Design review of the part shown in the three views and the two pictorial views. Dimensions are in mm from the part's minimum x, y and z. Coordinates: 2 decimals unless noted, no trailing zeros. Write each loop counter-clockwise with the first axis right and the second up, starting at its lowest first coordinate (ties: lowest second). Pieces come first, ordered by that corner, then holes. Notation, with made-up numbers: (81, 12.5) - (125, 12.5) arc R26 cw to (125, 51.5) - close; hole circle Ø2 at (31, 11.5). An arc over 180 degrees is marked (long way). Return JSON: item names as keys, results as strings. Group by question number.
(1) We need section D-D on y = 76. State the section outline as (x, z) points.
(2) Draft analysis for pull direction X (two halves, no side actions). For the marked faces 1, 2 and 3, state which applies: released by +X, released by -X, zero draft, split by the parting line, or undercut.
(3) For pin 1 Ø17.5 at (x, y) = (44.5, 55) entering from +Z; pin 2 Ø1.5 at (y, z) = (42, 2.5) entering from -X; pin 3 Ø5 at (y, z) = (69, 8.5) entering from +X (1 decimal); pin 4 Ø1.5 at (y, z) = (68, 2) entering from +X, all flat-tipped, find the tip position at first contact; note any pin that passes through.
(4) To check wall thickness, follow L1, parallel to Y at x = 44.45, z = 17.2 (1 decimal); L2, parallel to Y at x = 44.45, z = 8.75; L3, parallel to X at y = 32, z = 15. State the ranges of each line that lie inside material, in increasing order. Write a range as from..to.
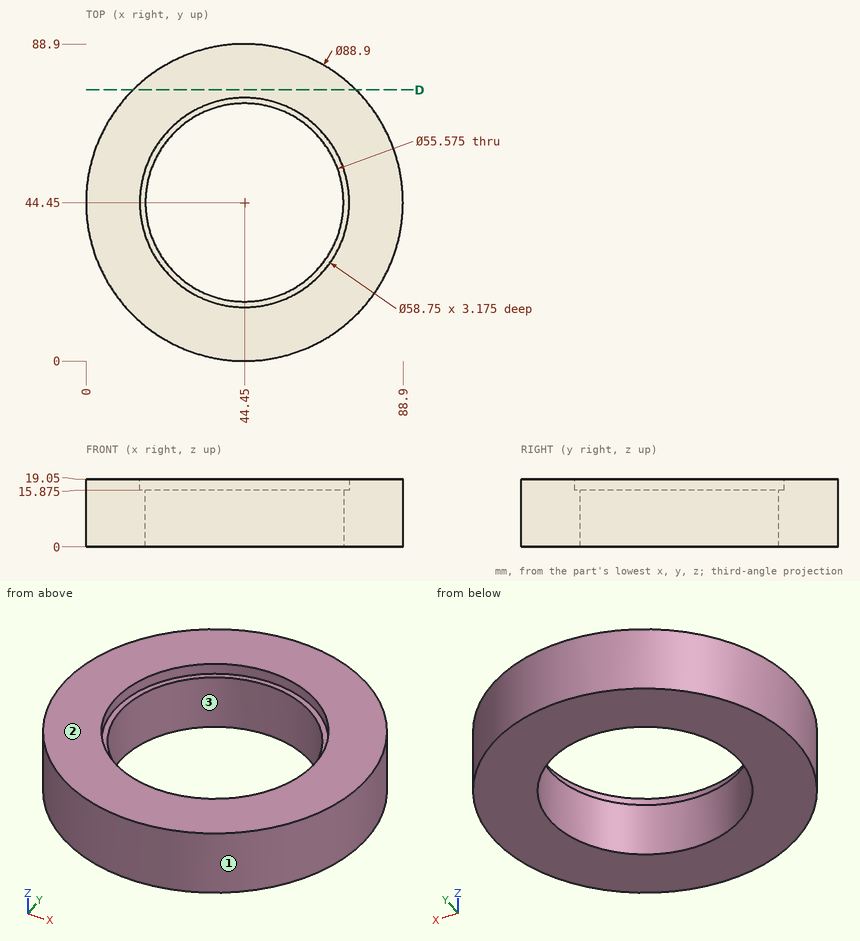
Ans:
{
 "1": {"outline": "(13.14, 0) - (75.76, 0) - (75.76, 19.05) - (13.14, 19.05) - close"},
 "2": {"face 1": "split by the parting line", "face 2": "zero draft", "face 3": "undercut"},
 "3": {"pin 1": "through", "pin 2": "x = 0.03", "pin 3": "x = 83", "pin 4": "x = 82.61"},
 "4": {"L1": "0..15.1, 73.8..88.9", "L2": "0..16.66, 72.24..88.9", "L3": "1.78..19.61, 69.29..87.12"}
}
